Source: CAD feature listing. Evaluate the final solid. Frame: model axes, mm. A direction names the side the tool comes from. Round coordinates to 2 decimals unless told otherwise and drop trailing zeros. Order: outer loops, then holes, each group sorted by start corner. A loop starts at its lowest first (then second) coordinate and runs counter-clockwise, first axis right, second up. Notation, with made-up numbers: M 39,-21.5 L 90,-21.5 A15 ccw 90,7.5 Z; hole C 87.25,89.25 d6. An arc over 180 degrees is marked long. Answer as CSV lines item,"result". Start each with the question number.
Item 1: Section query C-C on z = -4. Return the cut outline in (x, y), plus the area to 3 significant figures.
Item 2: Section query A-A on z = 16. Return the cut outline in (x, y).
Item 3: Line query: line 1 (Z direction, x = -5.9, y = 7); line 2 (Z direction, x = 29.5, y = 22.6); line 3 (X direction, y = 8.5, z = 37). Output: solid intervals per line, ascending. Write a range as [from, to].
Item 4: Set-up query: faces 1 (the face through (-3, 11, 39)), 2 (the face through (-4, 6, 20.75)), 3 (the face through (-6.1, 8.6, 23.3)). Return all of +Z, -Z, +X, -X, +Y, -Y with unobstructed straight access to the full face (end or side cutting, diameter ignored); none if empty.
Item 5: First-contact query: P1, Ø10, axis at x = 30.5, z = 12.5, coming from the -Y side; P2, Ø1, axis at y = 23, z = 27, coming from the -X side; P3, Ø6.5, axis at y = 7, z = 24.5, coming from the +X side; P4, Ø1.5, axis at y = 15.5, z = 7, coming from the +X side. Flat tips, straight axial feed; report the tip coordinate or a pass-through.
Item 6: Pull-direction query (Z, two-part tool) for faces 4 (the face through (-6.137, 7.434, 31.548)), 5 (the face through (42.5, 23, 29)), 6 (the face through (29.6, 20, -8.5)); classes: +Z half, -Z half, draft (parallel to the pull), parting line (faces both ways), or undercut.
Item 7: Section query B-B on y = 6.5. State how many separate pieces and enclosed holes the cut face has, plus the area to 3 significant figures.
from build123d import *

# Parameters (mm, degrees)
BOSS_EXTRU_1_DEPTH      = 58
ESQUISSE16_R            = 2
BOSS_EXTRU_2_DEPTH      = 4
ESQUISSE9_R             = 2
ENL_V_MAT_EXTRU_5_DEPTH = 10
ESQUISSE14_W            = 20
ESQUISSE14_H            = 19
ENL_V_MAT_EXTRU_7_DEPTH = 84.798866341
ESQUISSE5_W             = 3.5
ESQUISSE5_H             = 7.5
ENL_V_MAT_EXTRU_3_DEPTH = 12
CONG_6_R                = 2
CONG_11_R               = 10
ESQUISSE15_W            = 72.69818271
ESQUISSE15_H            = 50
ENL_V_MAT_EXTRU_8_DEPTH = 18
ESQUISSE17_R            = 8.5
ENL_V_MAT_EXTRU_9_DEPTH = 10
CHANFREIN1_SIZE         = 9
CHANFREIN1_SIZE2        = 6.538882752
CHANFREIN2_SIZE         = 5
CHANFREIN2_SIZE2        = 3.63271264
CONG_14_R               = 5
CONG_16_START           = 18
CONG_16_DEPTH           = 22
BOSS_EXTRU_3_START      = 2
BOSS_EXTRU_3_DEPTH      = 2
CONG_17_START           = 22
CONG_17_DEPTH           = 3


with BuildPart() as part:
    # Esquisse1 → Boss.-Extru.1 (new body)
    with BuildSketch(Plane.XY):
        Polygon((0, 0), (0, 18), (15, 18), (15, 0), (19, 0), (19, 18), (46, 18), (46, 22), (-7, 22), (-7, 0), align=None)
    extrude(amount=BOSS_EXTRU_1_DEPTH)

    # Esquisse16 → Boss.-Extru.2 (add)
    # profile 1 of 2: a face of its own
    with BuildSketch(Plane(origin=(0, 22, 0), x_dir=(1, 0, 0), z_dir=(0, 1, 0))):
        with BuildLine():
            Line((17, -3), (42, -3))
            Line((42, -3), (42, 0))
            Line((42, 0), (39.807764064, 0))
            ThreePointArc((39.807764064, 0), (35.990510002, 1.370899501), (33.91761317, 4.857142857))
            ThreePointArc((33.91761317, 4.857142857), (29.5, 8.5), (25.08238683, 4.857142857))
            ThreePointArc((25.08238683, 4.857142857), (23.009489998, 1.370899501), (19.192235936, 0))
            Line((19.192235936, 0), (17, 0))
            Line((17, 0), (17, -3))
        make_face()
        with Locations(Location((29.5, 4, 0), (0, 0, 270))):
            Circle(ESQUISSE16_R, mode=Mode.SUBTRACT)
    # profile 2 of 2: a face of its own
    with BuildSketch(Plane(origin=(0, 22, 0), x_dir=(1, 0, 0), z_dir=(0, 1, 0))):
        with BuildLine():
            Line((17, -58), (17, -55))
            Line((17, -55), (42, -55))
            Line((42, -55), (42, -58))
            Line((42, -58), (39.807764064, -58))
            ThreePointArc((39.807764064, -58), (35.990510002, -59.370899501), (33.91761317, -62.857142857))
            ThreePointArc((33.91761317, -62.857142857), (29.5, -66.5), (25.08238683, -62.857142857))
            ThreePointArc((25.08238683, -62.857142857), (23.009489998, -59.370899501), (19.192235936, -58))
            Line((19.192235936, -58), (17, -58))
        make_face()
        with Locations(Location((29.5, -62, 0), (0, 0, 270))):
            Circle(ESQUISSE16_R, mode=Mode.SUBTRACT)
    extrude(amount=-BOSS_EXTRU_2_DEPTH)

    # Esquisse9 → Enlèv. mat.-Extru.5 (cut)
    with BuildSketch(Plane.ZY.offset(7)):
        with Locations(Location((33.5, 7, 0), (0, 0, 270))):
            Circle(ESQUISSE9_R)
        with Locations(Location((24.5, 7, 0), (0, 0, 270))):
            Circle(ESQUISSE9_R)
    extrude(amount=-ENL_V_MAT_EXTRU_5_DEPTH, mode=Mode.SUBTRACT)

    # Esquisse14 → Enlèv. mat.-Extru.7 (cut, through all)
    with BuildSketch(Plane(origin=(0, 22, 0), x_dir=(1, 0, 0), z_dir=(0, 1, 0))):
        with Locations((3, -9.5)):
            Rectangle(ESQUISSE14_W, ESQUISSE14_H)
        with Locations((3, -48.5)):
            Rectangle(ESQUISSE14_W, ESQUISSE14_H)
    extrude(amount=-ENL_V_MAT_EXTRU_7_DEPTH, mode=Mode.SUBTRACT)

    # Esquisse5 → Enlèv. mat.-Extru.3 (cut)
    with BuildSketch(Plane.XZ):
        with Locations((-3.5, 33.5)):
            Rectangle(ESQUISSE5_W, ESQUISSE5_H)
        with Locations((-3.5, 24.5)):
            Rectangle(ESQUISSE5_W, ESQUISSE5_H)
    extrude(amount=-ENL_V_MAT_EXTRU_3_DEPTH, mode=Mode.SUBTRACT)

    # Congé6
    cong_6_edges = [part.edges().sort_by_distance(p)[0] for p in [
        (46, 20, 0),
        (46, 20, 58),
        (13, 20, 0),
        (13, 20, 58),
    ]]
    fillet(cong_6_edges, radius=CONG_6_R)

    # Congé11
    cong_11_edges = [part.edges().sort_by_distance(p)[0] for p in [
        (13, 20, 19),
        (13, 20, 39),
    ]]
    fillet(cong_11_edges, radius=CONG_11_R)

    # Esquisse15 → Enlèv. mat.-Extru.8 (cut)
    with BuildSketch(Plane.XZ):
        with Locations((29.349091355, -6)):
            Rectangle(ESQUISSE15_W, ESQUISSE15_H)
        with Locations((29.349091355, 64)):
            Rectangle(ESQUISSE15_W, ESQUISSE15_H)
    extrude(amount=-ENL_V_MAT_EXTRU_8_DEPTH, mode=Mode.SUBTRACT)

    # Esquisse17 → Enlèv. mat.-Extru.9 (cut)
    with BuildSketch(Plane(origin=(0, 22, 0), x_dir=(1, 0, 0), z_dir=(0, 1, 0))):
        with Locations(Location((29.5, -18, 0), (0, 0, 270))):
            Circle(ESQUISSE17_R)
        with Locations(Location((29.5, -40, 0), (0, 0, 270))):
            Circle(ESQUISSE17_R)
    extrude(amount=-ENL_V_MAT_EXTRU_9_DEPTH, mode=Mode.SUBTRACT)

    # Chanfrein1
    chanfrein1_edges = [part.edges().sort_by_distance(p)[0] for p in [
        (-7, 22, 29),
    ]]
    chanfrein1_side = [part.faces().sort_by_distance(p)[0] for p in [
        (-7, 11.242320797, 29),
    ]]
    chamfer(chanfrein1_edges, length=CHANFREIN1_SIZE, length2=CHANFREIN1_SIZE2, reference=chanfrein1_side[0])

    # Chanfrein2
    chanfrein2_edges = [part.edges().sort_by_distance(p)[0] for p in [
        (0, 18, 29),
    ]]
    chanfrein2_side = [part.faces().sort_by_distance(p)[0] for p in [
        (0, 9.150105695, 29),
    ]]
    chamfer(chanfrein2_edges, length=CHANFREIN2_SIZE, length2=CHANFREIN2_SIZE2, reference=chanfrein2_side[0])

    # Congé14
    cong_14_edges = [part.edges().sort_by_distance(p)[0] for p in [
        (3.63271264, 18, 29),
        (0, 13, 29),
    ]]
    fillet(cong_14_edges, radius=CONG_14_R)

    # Congé15
    # a fillet whose section is not a circle: 8, 6 mm, written as the material it takes off along each edge
    with BuildSketch(Plane(origin=(-0.461117248, 22, 5.17677837), x_dir=(1, 0, 0), z_dir=(0, 0, 1))) as cong_15_piece_1:
        with BuildLine():
            Bezier((1.604067641, 0), (0, 0), (-3.250034325, -4.473288486), weights=[1, 0.891006524, 1])
            Line((-3.250034325, -4.473288486), (0, 0))
            Line((0, 0), (1.604067641, 0))
        make_face()
    extrude(amount=47.64644326, mode=Mode.SUBTRACT)

    # Congé16: read off the stored shape, not the designer's step
    # Congé16 outline → Congé16 (cut)
    with BuildSketch(Plane.XY.offset(CONG_16_START)):
        with BuildLine():
            Line((-7, 13), (-7, 10.075722734))
            add(Edge.make_bspline(
                [(-7, 10.075722734), (-7, 13), (-5.281152949, 15.365790005)],
                knots=[0, 0, 0, 1, 1, 1], degree=2, weights=[1, 0.951056516, 1]))
            Line((-5.281152949, 15.365790005), (-7, 13))
        make_face()
    extrude(amount=CONG_16_DEPTH, mode=Mode.SUBTRACT)

    # Esquisse19 → Boss.-Extru.3 (add)
    with BuildSketch(Plane(origin=(0, 22, 0), x_dir=(1, 0, 0), z_dir=(0, 1, 0)).offset(BOSS_EXTRU_3_START)):
        with BuildLine():
            ThreePointArc((38, -18), (32.759601203, -25.850159234), (23.5, -24.020797289))
            Line((23.5, -24.020797289), (23.5, -33.979202711))
            ThreePointArc((23.5, -33.979202711), (32.759601203, -32.149840766), (38, -40))
            ThreePointArc((38, -40), (26.570520177, -47.979232292), (23.019259302, -34.5))
            Line((23.019259302, -34.5), (17, -34.5))
            ThreePointArc((17, -34.5), (16.646446609, -34.646446609), (16.5, -35))
            Line((16.5, -35), (16.5, -54))
            ThreePointArc((16.5, -54), (16.646446609, -54.353553391), (17, -54.5))
            Line((17, -54.5), (42, -54.5))
            ThreePointArc((42, -54.5), (42.353553391, -54.353553391), (42.5, -54))
            Line((42.5, -54), (42.5, -4))
            ThreePointArc((42.5, -4), (42.353553391, -3.646446609), (42, -3.5))
            Line((42, -3.5), (17, -3.5))
            ThreePointArc((17, -3.5), (16.646446609, -3.646446609), (16.5, -4))
            Line((16.5, -4), (16.5, -23))
            ThreePointArc((16.5, -23), (16.646446609, -23.353553391), (17, -23.5))
            Line((17, -23.5), (23.019259302, -23.5))
            ThreePointArc((23.019259302, -23.5), (26.570520177, -10.020767708), (38, -18))
        make_face()
    extrude(amount=-BOSS_EXTRU_3_DEPTH)

    # Congé17: read off the stored shape, not the designer's step
    # Congé17 outline → Congé17 (cut)
    with BuildSketch(Plane(origin=(0, 0, 0), x_dir=(1, 0, 0), z_dir=(0, 1, 0)).offset(CONG_17_START)):
        with BuildLine():
            ThreePointArc((23.668604651, -33.815759684), (23.560379709, -33.834820214), (23.5, -33.743003916))
            Line((23.5, -33.743003916), (23.5, -33.979202711))
            ThreePointArc((23.5, -33.979202711), (23.583737888, -33.896898934), (23.668604651, -33.815759684))
        make_face()
        with BuildLine():
            ThreePointArc((22.884548627, -23.337209302), (22.896939159, -23.443133109), (22.806719788, -23.5))
            Line((22.806719788, -23.5), (23.019259302, -23.5))
            ThreePointArc((23.019259302, -23.5), (22.951398096, -23.419023261), (22.884548627, -23.337209302))
        make_face()
        with BuildLine():
            ThreePointArc((23.668604651, -24.184240316), (23.583737888, -24.103101066), (23.5, -24.020797289))
            Line((23.5, -24.020797289), (23.5, -24.256996084))
            ThreePointArc((23.5, -24.256996084), (23.560379709, -24.165179786), (23.668604651, -24.184240316))
        make_face()
        with BuildLine():
            ThreePointArc((22.884548627, -34.662790698), (22.951398096, -34.580976739), (23.019259302, -34.5))
            Line((23.019259302, -34.5), (22.806719788, -34.5))
            ThreePointArc((22.806719788, -34.5), (22.896939159, -34.556866891), (22.884548627, -34.662790698))
        make_face()
    extrude(amount=CONG_17_DEPTH, mode=Mode.SUBTRACT)


solid = part.part
Results:
1,outline,"M 24.85,18 L 27.5,18 L 27.5,22 L 24.85,22 Z; M 31.5,18 L 34.15,18 L 34.15,22 L 31.5,22 Z"
1,area,"21.2 mm^2"
2,outline,"M 10.14,18 L 21.24,18 L 21.24,24 L 16.5,24 L 16.5,22 L 10.14,22 Z; M 37.76,18 L 46,18 L 46,22 L 42.5,22 L 42.5,24 L 37.76,24 Z"
3,line 1,"[19, 22.5], [26.5, 31.5], [35.5, 39]"
3,line 2,"[3.5, 9.5], [26.5, 31.5], [48.5, 54.5]"
3,line 3,"[-7, -5.25], [-1.75, 0], [15, 19]"
4,face 1,"+Z, -X, +Y, -Y"
4,face 2,"-Y"
4,face 3,"-X"
5,P1,"y = 18"
5,P2,"x = 23.5"
5,P3,"x = 19"
5,P4,"through"
6,face 4,"undercut"
6,face 5,"draft"
6,face 6,"-Z half"
7,separate pieces,"4"
7,enclosed holes,"0"
7,area,"140 mm^2"
